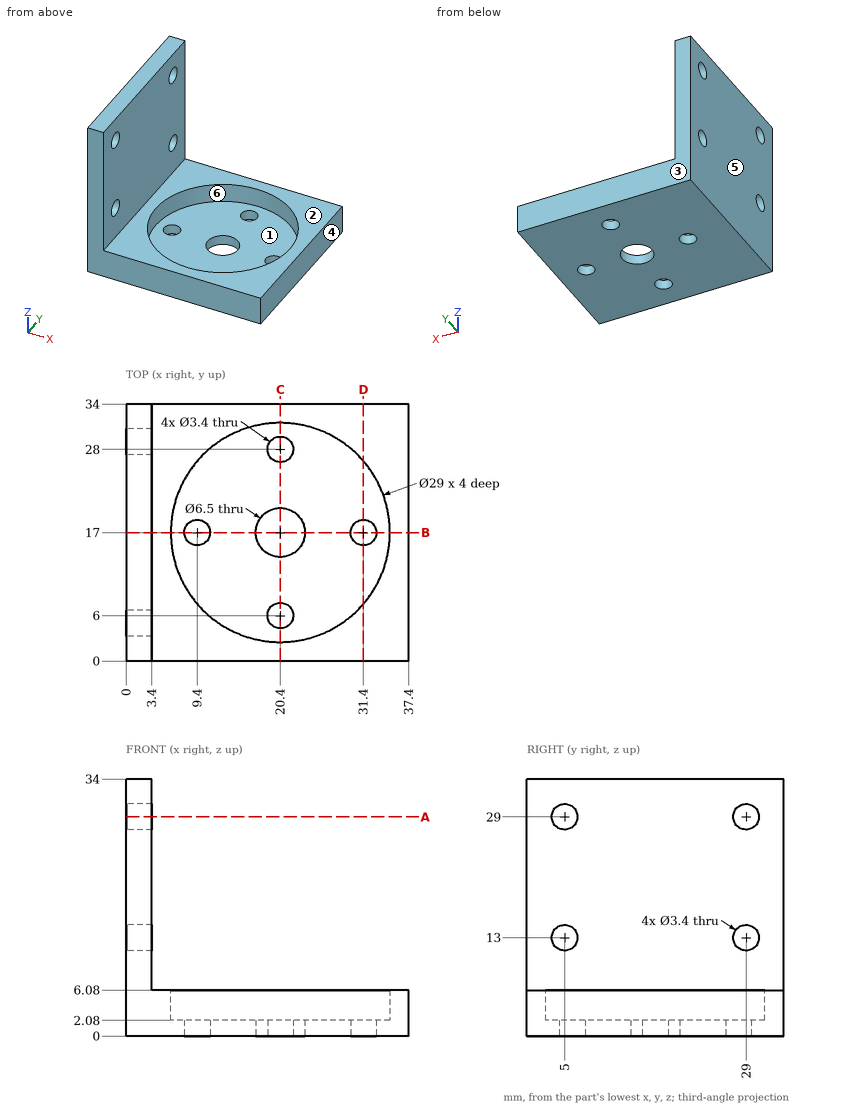
Check sheet for the drawn part. Datum: minimum x, y, z corner. Units: mm. A direction names the side the tool comes from. Coordinates: 2 decimals unless noted, no trailing zeros. Order: outer loops, then holes, each group sorted by start corner. A loop starts at its lowest first (then second) coordinate and runs counter-clockwise, first axis right, second up. Notation, with made-up numbers: (-19, 83.25) -> (19, 83.25) arc R28 ccw to (19, 108.25) -> close; hole circle Ø11 at (86, -11). An arc over 180 degrees is marked (long way). Write each question's results on one line, items separated by ' | '. Start each with the question number.
1) Section check B-B (y = 17). Enter the section's corners in (x, z).
2) Material ranges on line 1 along X through (y, z) = (17, 0.6); line 2 along Z through (x, y) = (2.3, 5); line 3 along Y through (x, z) = (20, 1), recorded low to high.
3) Section check A-A (z = 29). Enter the section's corners in (x, y), and give its area (3 significant figures).
4) Section check C-C (x = 20.4). Enter the section's corners in (y, z).
5) Section check D-D (x = 31.4). Enter the section's corners in (y, z), and give its area (3 significant figures).
6) Depth check by flat-ended pin: pin 1 (2 mm diameter, centred on y = 10.5, z = 11, fed in from -X); pin 2 (4 mm diameter, centred on x = 9.4, y = 17, fed in from +Z); pin 3 (4.5 mm diameter, centred on y = 29, z = 13, fed in from +X); pin 4 (17 mm diameter, centred on x = 25.5, y = 25, fed in from +Z). Enter the tip coordinate at first touch or a pass-through.
7) Set-up check for the marked faces 1, 2 and 3: record each of +Z, -Z, +X, -X, +Y, -Y from which the full face is reachable in a straight line by a thin tool's end or side.
8) Draft check along X on the marked faces 4, 5 and 6. Enter one of: pulls with the +X half, pulls with the -X half, needs draft (parallel to the pull), parting line crosses it, or undercut.
Checked values:
1) outline: (0, 0) -> (7.7, 0) -> (7.7, 2.08) -> (5.9, 2.08) -> (5.9, 6.08) -> (3.4, 6.08) -> (3.4, 34) -> (0, 34) -> close; (11.1, 0) -> (17.15, 0) -> (17.15, 2.08) -> (11.1, 2.08) -> close; (23.65, 0) -> (29.7, 0) -> (29.7, 2.08) -> (23.65, 2.08) -> close; (33.1, 0) -> (37.4, 0) -> (37.4, 6.08) -> (34.9, 6.08) -> (34.9, 2.08) -> (33.1, 2.08) -> close
2) line 1: 0 to 7.7, 11.1 to 17.15, 23.65 to 29.7, 33.1 to 37.4 | line 2: 0 to 11.3, 14.7 to 27.3, 30.7 to 34 | line 3: 0 to 4.35, 7.65 to 13.77, 20.23 to 26.35, 29.65 to 34
3) outline: (0, 0) -> (3.4, 0) -> (3.4, 3.3) -> (0, 3.3) -> close; (0, 6.7) -> (3.4, 6.7) -> (3.4, 27.3) -> (0, 27.3) -> close; (0, 30.7) -> (3.4, 30.7) -> (3.4, 34) -> (0, 34) -> close | area: 92.5 mm²
4) outline: (0, 0) -> (4.3, 0) -> (4.3, 2.08) -> (2.5, 2.08) -> (2.5, 6.08) -> (0, 6.08) -> close; (7.7, 0) -> (13.75, 0) -> (13.75, 2.08) -> (7.7, 2.08) -> close; (20.25, 0) -> (26.3, 0) -> (26.3, 2.08) -> (20.25, 2.08) -> close; (29.7, 0) -> (34, 0) -> (34, 6.08) -> (31.5, 6.08) -> (31.5, 2.08) -> (29.7, 2.08) -> close
5) outline: (0, 0) -> (15.3, 0) -> (15.3, 2.08) -> (7.55, 2.08) -> (7.55, 6.08) -> (0, 6.08) -> close; (18.7, 0) -> (34, 0) -> (34, 6.08) -> (26.45, 6.08) -> (26.45, 2.08) -> (18.7, 2.08) -> close | area: 124 mm²
6) pin 1: x = 0 | pin 2: z = 2.08 | pin 3: x = 3.4 | pin 4: z = 6.08
7) face 1: +Z | face 2: +Z, +X, +Y, -Y | face 3: +Z, -Z, +X, -X, +Y
8) face 4: pulls with the +X half | face 5: pulls with the -X half | face 6: undercut
